```python
from build123d import *

# Parameters (mm, degrees)
SKETCH1_W           = 200
SKETCH1_H           = 200
BOSS_EXTRUDE1_DEPTH = 76.2
SKETCH2_W           = 180
SKETCH2_H           = 180
CUT_EXTRUDE2_DEPTH  = 80
SKETCH3_W           = 180
SKETCH3_H           = 180
BOSS_EXTRUDE2_DEPTH = 10


with BuildPart() as part:
    # Sketch1 → Boss-Extrude1 (new body)
    with BuildSketch(Plane.XY):
        with Locations((-100, 100)):
            Rectangle(SKETCH1_W, SKETCH1_H)
    extrude(amount=BOSS_EXTRUDE1_DEPTH)

    # Sketch2 → Cut-Extrude2 (cut)
    with BuildSketch(Plane.XY.offset(76.2)):
        with Locations((-100, 100)):
            Rectangle(SKETCH2_W, SKETCH2_H)
    extrude(amount=-CUT_EXTRUDE2_DEPTH, mode=Mode.SUBTRACT)

    # Sketch3 → Boss-Extrude2 (add)
    with BuildSketch(Plane.XY):
        with Locations((-100, 100)):
            Rectangle(SKETCH3_W, SKETCH3_H)
    extrude(amount=BOSS_EXTRUDE2_DEPTH)


solid = part.part
```
Geometry: final body of the model. Coordinates: model frame, mm. A direction names the side the tool comes from. Round coordinates to 2 decimals unless told otherwise and drop trailing zeros. Loops run counter-clockwise (first coordinate to the right, second up) from the corner with the lowest first, then second, coordinate; pieces in that order, holes last. Notation, with made-up numbers: (71, 86) -> (98, 86) arc R24 cw to (98, 118) -> close; hole circle Ø9 at (-1.75, -35.75). An arc over 180 degrees is marked (long way). Use one line per item in the form item = value. Start each with the question number.
1) Section A-A on z = 24. Output: boundary loops of the cut face in (x, y).
2) Draft query along X for faces 1 (the flat face through (-101, 200, 38)), 2 (the flat face through (-200, 99, 38)), 3 (the flat face through (-101, 190, 44)). Return one class per face: released by +X, released by -X, zero draft, split by the parting line, or undercut.
3) First-contact query: P1, Ø10, axis at x = -61, y = 69.5, coming from the +Z side. Flat tip, straight axial feed; report the tip coordinate or a pass-through.
4) Section B-B on y = 94. Output: boundary loops of the cut face in (x, z), then the cut area to 3 significant figures.
5) Section C-C on x = -105.5. Output: boundary loops of the cut face in (y, z).
6) Line query: L1, parallel to X at y = 188, z = 11; L2, parallel to Y at x = -111, z = 34; L3, parallel to Z at x = -145, y = 48.5. Output: solid intervals per line, ascending.
7) Access query for faces 4 (the flat face through (-190, 99, 44)), 5 (the flat face through (-101, 0, 38)). Directions: +Z, -Z, +X, -X, +Y, -Y. A direction counts if a zero-diameter tool reaches every point of the face in a straight line with its end or side. Return the directions, or none.
Response:
q1.outline = (-200, 0) -> (0, 0) -> (0, 200) -> (-200, 200) -> close; hole (-190, 10) -> (-10, 10) -> (-10, 190) -> (-190, 190) -> close
q2.face_1 = zero draft
q2.face_2 = released by -X
q2.face_3 = undercut
q3.P1 = 10
q4.outline = (-200, 0) -> (0, 0) -> (0, 76.2) -> (-10, 76.2) -> (-10, 10) -> (-190, 10) -> (-190, 76.2) -> (-200, 76.2) -> close
q4.area = 3,320 mm^2
q5.outline = (0, 0) -> (200, 0) -> (200, 76.2) -> (190, 76.2) -> (190, 10) -> (10, 10) -> (10, 76.2) -> (0, 76.2) -> close
q6.L1 = -200 to -190, -10 to 0
q6.L2 = 0 to 10, 190 to 200
q6.L3 = 0 to 10
q7.face_4 = +Z
q7.face_5 = +Z, -Z, +X, -X, -Y
